Input: dimensioned drawing with shaded views. Units: mm. Origin: part minimum x, y, z. Give positions to 0.01 mm unless a question says otherwise; leave off trailing zeros. Order: outer loops, then holes, each group sorted by start corner. A loop starts at its lowest first (then second) coordinate and runs counter-clockwise, first axis right, second up. Notation, with made-up numbers: (-20.75, 34.5) - (35.25, 34.5) arc R14 ccw to (35.25, 50.5) - close; hole circle Ø3 at (8.25, 4.5). An arc over 180 degrees is marked (long way). Answer as CSV lines item,"result".
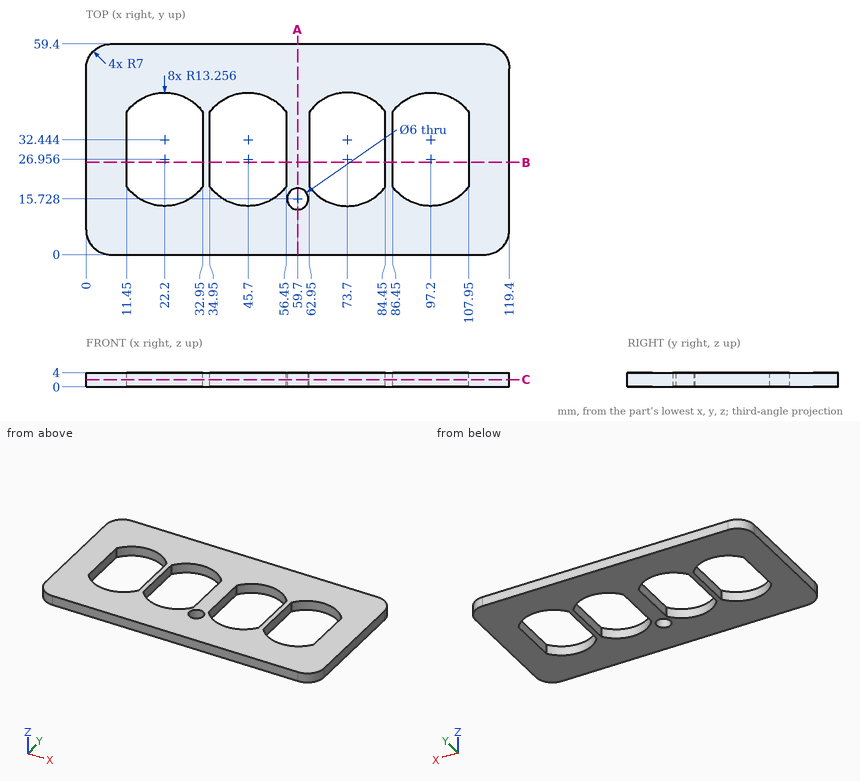
(1) Cut plane B-B (y = 26). Return loops of the section in (x, z).
Completed:
outline,"(0, 0) - (11.45, 0) - (11.45, 4) - (0, 4) - close; (32.95, 0) - (34.95, 0) - (34.95, 4) - (32.95, 4) - close; (56.45, 0) - (62.95, 0) - (62.95, 4) - (56.45, 4) - close; (84.45, 0) - (86.45, 0) - (86.45, 4) - (84.45, 4) - close; (107.95, 0) - (119.4, 0) - (119.4, 4) - (107.95, 4) - close"
(2) Cut plane C-C (z = 2). Return loops of the section in (x, y).
Completed:
outline,"(0, 7) arc R7 ccw to (7, 0) - (112.4, 0) arc R7 ccw to (119.4, 7) - (119.4, 52.4) arc R7 ccw to (112.4, 59.4) - (7, 59.4) arc R7 ccw to (0, 52.4) - close; hole (11.45, 19.2) arc R13.26 ccw to (32.95, 19.2) - (32.95, 40.2) arc R13.26 ccw to (11.45, 40.2) - close; hole (34.95, 19.2) arc R13.26 ccw to (56.45, 19.2) - (56.45, 40.2) arc R13.26 ccw to (34.95, 40.2) - close; hole circle Ø6 at (59.7, 15.73); hole (62.95, 19.2) arc R13.26 ccw to (84.45, 19.2) - (84.45, 40.2) arc R13.26 ccw to (62.95, 40.2) - close; hole (86.45, 19.2) arc R13.26 ccw to (107.95, 19.2) - (107.95, 40.2) arc R13.26 ccw to (86.45, 40.2) - close"
(3) Cut plane A-A (x = 59.7). Return loops of the section in (y, z), then the cut area to 3 significant figures.
Completed:
outline,"(0, 0) - (12.73, 0) - (12.73, 4) - (0, 4) - close; (18.73, 0) - (59.4, 0) - (59.4, 4) - (18.73, 4) - close"
area,"214 mm²"
(4) Ray query, line 1 (X direction, y = 38, z = 1.4); line 2 (Y direction, x = 59.7, z = 1.85); line 3 (Y direction, x = 97.5, z = 1.2). Return the intervals inside material, ascending. Write a range as from..to.
Completed:
line 1,"0..11.45, 32.95..34.95, 56.45..62.95, 84.45..86.45, 107.95..119.4"
line 2,"0..12.73, 18.73..59.4"
line 3,"0..13.7, 45.7..59.4"
